```python
from build123d import *

# Parameters (mm, degrees)
F1_DEPTH = 124.46
F3_D     = 4.4958
F5_D     = 3.2639


with BuildPart() as f1:
    # F0 (on Front) → F1 (new body)
    with BuildSketch(Plane.XZ):
        with BuildLine():
            Line((0, 21.3614), (0, 0))
            Line((0, 0), (2.0574, 0))
            Line((2.0574, 0), (2.0574, 21.3614))
            ThreePointArc((2.0574, 21.3614), (3.4560236985, 24.7379763015), (6.8326, 26.1366))
            Line((6.8326, 26.1366), (174.1424, 26.1366))
            ThreePointArc((174.1424, 26.1366), (177.5189763015, 24.7379763015), (178.9176, 21.3614))
            Line((178.9176, 21.3614), (178.9176, 0))
            Line((178.9176, 0), (180.975, 0))
            Line((180.975, 0), (180.975, 21.3614))
            ThreePointArc((180.975, 21.3614), (178.9737777931, 26.1927777931), (174.1424, 28.194))
            Line((174.1424, 28.194), (6.8326, 28.194))
            ThreePointArc((6.8326, 28.194), (2.0012222069, 26.1927777931), (0, 21.3614))
        make_face()
    extrude(amount=-F1_DEPTH)

    # F3 (through all)
    with Locations(Plane.YZ.offset(180.975)):
        with Locations((19.3675, 7.9502), (105.0925, 7.9502)):
            Hole(F3_D / 2)

    # F5 (through all)
    with Locations(Plane(origin=(0, 0, 26.1366), x_dir=(1, 0, 0), z_dir=(0, 0, -1))):
        with Locations((14.2875, -16.51), (14.2875, -107.95), (166.6875, -16.51), (166.6875, -107.95)):
            Hole(F5_D / 2)


solid = f1.part
```
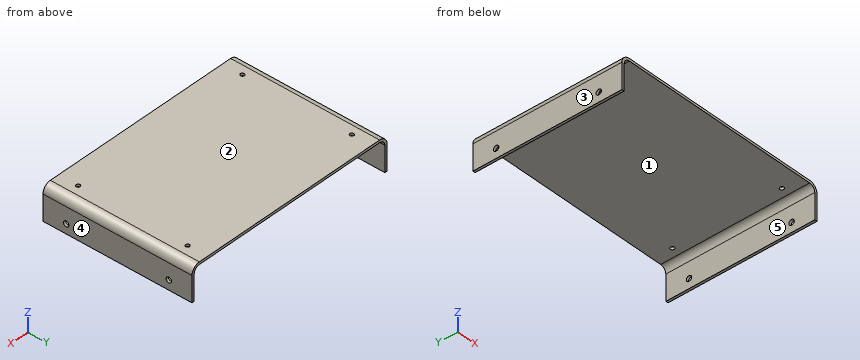
Geometry check sheet. Reference: the model listing, model coordinates, mm. Face numbers are marked on the shaded views. A direction names the side the tool comes from. Coordinates: 2 decimals unless noted, no trailing zeros. Loops run counter-clockwise (first coordinate to the right, second up) from the corner with the lowest first, then second, coordinate; pieces in that order, holes last. Notation, with made-up numbers: (78.5, 14.25) - (100.5, 14.25) arc R20 ccw to (100.5, 51.25) - close; hole circle Ø4 at (78, 1.25). An arc over 180 degrees is marked (long way). One line per item, written item: value. Start each with the question number.
(1) Cross-section at B-B on y = 28. Enter the section's corners in (x, z) (3 decimals), plus the area to 3 significant figures.
(2) Tool access check on the marked faces 1 and 2. Record the directions out of +Z, -Z, +X, -X, +Y, -Y that give a thin tool (end or side, any length) a straight path to the whole face; none if there is none.
(3) Material ranges on line 1 (X direction, y = 27.5, z = 6.5) (3 decimals); line 2 (X direction, y = 16.51, z = 26.75); line 3 (Z direction, x = 167.5, y = 110), recorded low to high. Write a range as [from, to].
(4) Cross-section at C-C on x = 65. Enter the section's corners in (y, z), plus the area to 3 significant figures.
(5) Depth check by flat-ended pin: P1, Ø5, axis at x = 166.69, y = 16.51, coming from the -Z side; P2, Ø1.5, axis at y = 21, z = 23, coming from the +X side. Enter the tip coordinate at first touch or a pass-through.
(6) Cross-section at A-A on z = 14. Enter the section's corners in (x, y) (3 decimals).
(7) Mould release check, pull along X, two halves, no side actions. Record for the marked faces 3, 4 and 5: released by +X, released by -X, zero draft, split by the parting line, or undercut.
Results below:
1. outline: (0, 0) - (2.057, 0) - (2.057, 21.361) arc R4.775 cw to (6.833, 26.137) - (174.142, 26.137) arc R4.775 cw to (178.918, 21.361) - (178.918, 0) - (180.975, 0) - (180.975, 21.361) arc R6.833 ccw to (174.142, 28.194) - (6.833, 28.194) arc R6.833 ccw to (0, 21.361) - close
1. area: 470 mm2
2. face 1: -Z, +Y, -Y
2. face 2: +Z, +X, -X, +Y, -Y
3. line 1: x = [0, 2.057], [178.918, 180.975]
3. line 2: x = [2.63, 12.66], [15.92, 165.06], [168.32, 178.34]
3. line 3: z = [26.14, 28.19]
4. outline: (0, 26.14) - (124.46, 26.14) - (124.46, 28.19) - (0, 28.19) - close
4. area: 256 mm2
5. P1: stops at z = 26.14
5. P2: stops at x = 180.92
6. outline: (0, 0) - (2.057, 0) - (2.057, 124.46) - (0, 124.46) - close; (178.918, 0) - (180.975, 0) - (180.975, 124.46) - (178.918, 124.46) - close
7. face 3: released by -X
7. face 4: released by +X
7. face 5: undercut
